Check sheet for the modelled part. Datum: model origin and axes. Units: mm. A direction names the side the tool comes from. Coordinates: 2 decimals unless noted, no trailing zeros. Order: outer loops, then holes, each group sorted by start corner. A loop starts at its lowest first (then second) coordinate and runs counter-clockwise, first axis right, second up.
from build123d import *

# Parameters (mm, degrees)
F0_W     = 31.75
F0_H     = 63.5
F1_DEPTH = 25.4
F4_D     = 12.7
F4_DEPTH = 25.4
F4_TIP   = 3.8154649308
F5_W     = 8.89
F5_H     = 8.89
F6_DEPTH = 25.4
F7_D     = 19.05
F7_DEPTH = 50.8
F7_TIP   = 5.7231973962


# Not quite as in the source:
# - a feature names something its author has since deleted; it is built from what else it names


with BuildPart() as f1:
    # F0 (on Front) → F1 (new body)
    with BuildSketch(Plane.XZ):
        with Locations((15.875, 31.75)):
            Rectangle(F0_W, F0_H)
        with Locations((-15.875, 31.75)):
            Rectangle(F0_W, F0_H)
    extrude(amount=-F1_DEPTH)

    # F4
    with Locations(Plane.XZ):
        with Locations((24.6206466109, 21.9729263335)):
            Hole(F4_D / 2, depth=F4_DEPTH)
            with Locations((0, 0, -(F4_DEPTH + F4_TIP / 2))):  # 118° drill point
                Cone(0, F4_D / 2, F4_TIP, mode=Mode.SUBTRACT)

    # F5 (on face) → F6 (join)
    with BuildSketch(Plane(origin=(0, 25.4, 0), x_dir=(-1, 0, 0), z_dir=(0, 1, 0))):
        with Locations((-27.305, 59.055)):
            Rectangle(F5_W, F5_H)
        with Locations((27.305, 59.055)):
            Rectangle(F5_W, F5_H)
        with Locations((-27.305, 4.445)):
            Rectangle(F5_W, F5_H)
        with Locations((27.305, 4.445)):
            Rectangle(F5_W, F5_H)
    extrude(amount=F6_DEPTH)

    # F7
    with Locations(Plane.XY.offset(63.5)):
        with Locations((-21.082, 12.1284499764), (0, 11.9907837361)):
            Hole(F7_D / 2, depth=F7_DEPTH)
            with Locations((0, 0, -(F7_DEPTH + F7_TIP / 2))):  # 118° drill point
                Cone(0, F7_D / 2, F7_TIP, mode=Mode.SUBTRACT)


solid = f1.part
(1) Release check for a two-part mould opening along X. For faces 6 (the flat face through (27, 38, 8.89)), 7 (the cylindrical face through (-13.523, 6.333, 37.744)), 8 (the flat face through (31.75, 19, 31)), 9 (the flat face through (0, 25.4, 32)) record: +X half, -X half, draft (parallel to the pull), parting line (faces both ways), or undercut.
Filled in:
face 6: draft
face 7: undercut
face 8: +X half
face 9: undercut
(2) Tool access check on faces 1 (the cylindrical face through (1.24, 21.435, 37.744)), 2 (the flat face through (-27, 38, 54.61)), 3 (the flat face through (-22.86, 38, 59)), 4 (the flat face through (0, 19, 0)), 5 (the flat face through (27, 50.8, 59)). Record the directions out of +Z, -Z, +X, -X, +Y, -Y that give a thin tool (end or side, any length) a straight path to the whole face; none if there is none.
Filled in:
face 1: +Z
face 2: +X, -X, +Y
face 3: +Z, -Z, +Y
face 4: -Z, +X, -X, +Y, -Y
face 5: +Z, -Z, +X, -X, +Y
(3) Cross-section at A-A (y = 32). Enter the section's corners in (x, z), and give its area (3 significant figures).
Filled in:
outline: (-31.75, 0) - (-22.86, 0) - (-22.86, 8.89) - (-31.75, 8.89) - close; (-31.75, 54.61) - (-22.86, 54.61) - (-22.86, 63.5) - (-31.75, 63.5) - close; (22.86, 0) - (31.75, 0) - (31.75, 8.89) - (22.86, 8.89) - close; (22.86, 54.61) - (31.75, 54.61) - (31.75, 63.5) - (22.86, 63.5) - close
area: 316 mm2
(4) Go/stop test with flat-tipped pins: P1, Ø10, axis at x = -10, z = 40, coming from the +Y side; P2, Ø11.5, axis at x = -21.08, y = 12.13, coming from the +Z side. Record where each tip stops, or that it passes through.
Filled in:
P1: stops at y = 25.4
P2: stops at z = 10.43
(5) Thickness scan on probe 1 along X at (y, z) = (7, 55); probe 2 along Y at (x, z) = (0, 43.5); probe 3 along X at (y, z) = (15, 33). Record the ranges inside material, lowest first.
Filled in:
probe 1: x = -31.75 to -29.11, -13.06 to -8.11, 8.11 to 31.75
probe 2: y = 0 to 2.47, 21.52 to 25.4
probe 3: x = -31.75 to -30.16, -12 to -9.04, 9.04 to 31.75
(6) Cross-section at C-C (z = 31.5). Enter the section's corners in (x, y) (3 decimals).
Filled in:
outline: (-31.75, 0) - (31.75, 0) - (31.75, 25.4) - (-31.75, 25.4) - close; hole circle Ø19.05 at (-21.082, 12.128); hole circle Ø19.05 at (0, 11.991)
(7) Cross-section at B-B (x = 26). Enter the section's corners in (y, z), and give its area (3 significant figures).
Filled in:
outline: (0, 0) - (50.8, 0) - (50.8, 8.89) - (25.4, 8.89) - (25.4, 15.77) - (0, 15.77) - close; (0, 28.17) - (25.4, 28.17) - (25.4, 54.61) - (50.8, 54.61) - (50.8, 63.5) - (0, 63.5) - close
area: 1,750 mm2
